```python
from build123d import *

# Parameters (mm, degrees)
SKETCH1_R           = 1.75
BOSS_EXTRUDE1_DEPTH = 2
SKETCH_1_R          = 2
CUT_EXTRUDE_1_DEPTH = 10


with BuildPart() as part:
    # Sketch1 → Boss-Extrude1 (new body)
    with BuildSketch(Plane.XY):
        with BuildLine():
            ThreePointArc((-0.413391137, 3.978581125), (-3.985278749, -0.34286046), (0.272222222, -3.990726132))
            ThreePointArc((0.272222222, -3.990726132), (29.90408025, -3.227529096), (59.494248826, -4.974355813))
            ThreePointArc((59.494248826, -4.974355813), (64.981597081, -0.428591321), (60.351328502, 4.987641555))
            ThreePointArc((60.351328502, 4.987641555), (29.947025925, 5.804484659), (-0.413391137, 3.978581125))
        make_face()
        Circle(SKETCH1_R, mode=Mode.SUBTRACT)
        with Locations((60, 0)):
            Circle(SKETCH1_R, mode=Mode.SUBTRACT)
    extrude(amount=BOSS_EXTRUDE1_DEPTH)

    # 草图1 → 切除-拉伸1 (cut)
    with BuildSketch(Plane.XY.offset(2)):
        with Locations((28.961050448, 1.261749932)):
            Circle(SKETCH_1_R)
    extrude(amount=-CUT_EXTRUDE_1_DEPTH, mode=Mode.SUBTRACT)


solid = part.part
```
The listing builds one solid part. Answer for the finished solid, in the listing's coordinates (mm). Round coordinates to 2 decimals unless told otherwise and drop trailing zeros. Write each loop counter-clockwise with the first axis right and the second up, starting at its lowest first coordinate (ties: lowest second). Pieces come first, ordered by that corner, then holes. Notation, with made-up numbers: (25, 78) -> (47, 78) arc R24 cw to (47, 115) -> close; hole circle Ø10 at (7.25, -4). An arc over 180 degrees is marked (long way). Use CSV: the item, a comma, the result in double quotes. Start each with the question number.
(1) Section C-C on x = 23.5 is taken. Give the vertices of the cut face in (y, z), then the cut area to 3 significant figures.
(2) The mould has two halves that part along X. Classify faces 1 (the face through (30, -1, 2)), 2 (the face through (30.37, 5.81, 0.99)), 3 (the face through (61.617, -0.67, 0.986)), 4 (the face through (29.49, -3.22, 0.99)): released by +X, released by -X, zero draft, split by the parting line, or undercut.
(3) Section B-B on y = 0 is taken. Give the vertices of the cut face in (x, z), then the cut area to 3 significant figures.
(4) Section A-A on z = 0.85 is taken. Give the vertices of the cut face in (x, y), then the cut area to 3 significant figures.
(5) Consider L1, parallel to Y at x = 60, z = 0.85; L2, parallel to Y at x = 0, z = 1.15; L3, parallel to X at y = -1.25, z = 1.15. Determine where each line is inside the solid, lowest interval first. Write a range as from..to.
A:
1,outline,"(-3.18, 0) -> (5.64, 0) -> (5.64, 2) -> (-3.18, 2) -> close"
1,area,"17.6 mm²"
2,face 1,"zero draft"
2,face 2,"split by the parting line"
2,face 3,"undercut"
2,face 4,"undercut"
3,outline,"(-4, 0) -> (-1.75, 0) -> (-1.75, 2) -> (-4, 2) -> close; (1.75, 0) -> (27.41, 0) -> (27.41, 2) -> (1.75, 2) -> close; (30.51, 0) -> (58.25, 0) -> (58.25, 2) -> (30.51, 2) -> close; (61.75, 0) -> (65, 0) -> (65, 2) -> (61.75, 2) -> close"
3,area,"118 mm²"
4,outline,"(-0.41, 3.98) arc R4 ccw to (0.27, -3.99) arc R350 cw to (59.49, -4.97) arc R5 ccw (long way) to (60.35, 4.99) arc R350 ccw to start; hole circle Ø3.5 at (0, 0); hole circle Ø4 at (28.96, 1.26); hole circle Ø3.5 at (60, 0)"
4,area,"575 mm²"
5,L1,"y = -5..-1.75, 1.75..5.01"
5,L2,"y = -4..-1.75, 1.75..4.02"
5,L3,"x = -3.8..-1.22, 1.22..58.78, 61.22..64.84"
